Could you check a few things on this drawing? It's one solid part, dimensions in mm from its lowest x, y, z. Round coordinates to 2 decimals unless told otherwise and drop trailing zeros. Write each loop counter-clockwise with the first axis right and the second up, starting at its lowest first coordinate (ties: lowest second). Pieces come first, ordered by that corner, then holes. Notation, with made-up numbers: (83, 34) - (119, 34) arc R5 ccw to (119, 39) - close; hole circle Ø10 at (19, -5.75). An arc over 180 degrees is marked (long way). Use one line per item in the form item = value. Start each with the question number.
1. If I drill on line 1 along Y through (x, z) = (23, 14.75); line 2 along X through (y, z) = (6.5, 23.25); line 3 along X through (y, z) = (7.5, 5.5) (1 decimal), over which ranges is the centre line in solid material (lowest first)?
2. Will these pins go through, and if not, where does the flat tip stop? pin 1 (6 mm diameter, centred on x = 15.5, z = 21.5, fed in from -Y) (1 decimal); pin 2 (2 mm diameter, centred on x = 31, z = 8.5, fed in from -Y); pin 3 (12 mm diameter, centred on x = 18.5, z = 12.5, fed in from +Y).
3. I want a section at B-B, the plane x = 30. List the corners of the cut face in (y, z) for me.
4. I want a section at A-A, the plane z = 17. List the corners of the cut face in (x, y) for me (1 decimal).
5. I want a section at C-C, the plane y = 38.5. List the corners of the cut face in (x, z) for me, plus the area to 3 significant figures.
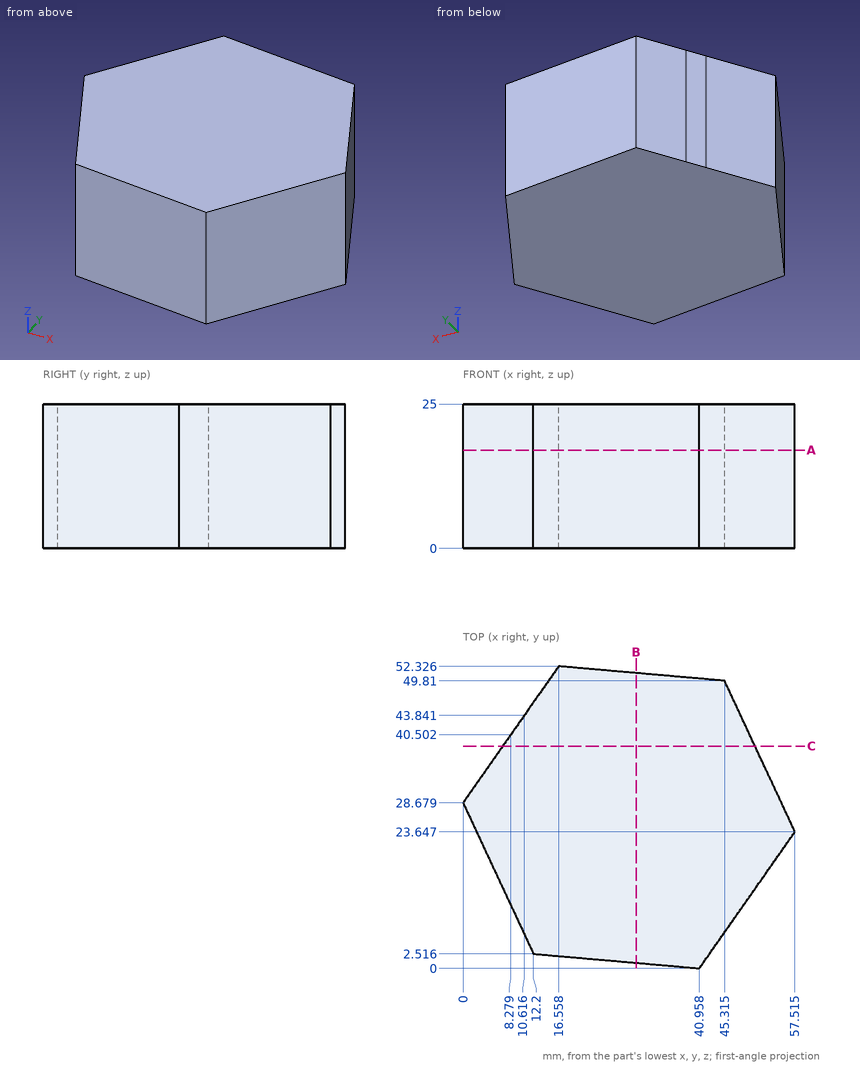
Model answer:
q1.line_1 = 1.57 to 51.76
q1.line_2 = 10.34 to 45.51
q1.line_3 = 9.9 to 46.2
q2.pin_1 = 2
q2.pin_2 = 0.78
q2.pin_3 = 52.33
q3.outline = (0.96, 0) - (51.15, 0) - (51.15, 25) - (0.96, 25) - close
q4.outline = (0, 28.7) - (12.2, 2.5) - (41, 0) - (57.5, 23.6) - (45.3, 49.8) - (16.6, 52.3) - close
q5.outline = (6.88, 0) - (50.59, 0) - (50.59, 25) - (6.88, 25) - close
q5.area = 1,090 mm2
